from build123d import *

# Parameters (mm, degrees)
SALIENTE_EXTRUIR2_DEPTH = 3
CROQUIS2_W              = 3
CROQUIS2_H              = 10
SALIENTE_EXTRUIR3_DEPTH = 3
CROQUIS3_W              = 10
CROQUIS3_H              = 3
SALIENTE_EXTRUIR4_DEPTH = 3


with BuildPart() as part:
    # Croquis1 → Saliente-Extruir2 (new body)
    with BuildSketch(Plane.XY):
        Polygon((19, -9), (-19, -9), (-19, 9), (-1.5, 9), (-1.5, 6), (-3, 6), (-3, 3), (3, 3), (3, 6), (1.5, 6), (1.5, 9), (19, 9), align=None)
    extrude(amount=SALIENTE_EXTRUIR2_DEPTH)

    # Croquis2 → Saliente-Extruir3 (add)
    with BuildSketch(Plane(origin=(19, 0, 0), x_dir=(0, 0, -1), z_dir=(1, 0, 0))):
        with Locations((-1.5, 0)):
            Rectangle(CROQUIS2_W, CROQUIS2_H)
    saliente_extruir3 = extrude(amount=SALIENTE_EXTRUIR3_DEPTH)

    # Croquis3 → Saliente-Extruir4 (add)
    with BuildSketch(Plane(origin=(0, 9, 0), x_dir=(1, 0, 0), z_dir=(0, 1, 0))):
        with Locations((14.325, -1.5)):
            Rectangle(CROQUIS3_W, CROQUIS3_H)
    saliente_extruir4 = extrude(amount=SALIENTE_EXTRUIR4_DEPTH)

    # Simetría1: Saliente-Extruir3 across plane
    add(saliente_extruir3.mirror(Plane(origin=(0, 0, 0), x_dir=(0, 0, 1), z_dir=(1, 0, 0))))

    # Simetría2: Saliente-Extruir4 across plane
    add(saliente_extruir4.mirror(Plane(origin=(0, 0, 0), x_dir=(0, 0, 1), z_dir=(1, 0, 0))))


solid = part.part
Read the model definition and answer for the solid it produces. Units are mm, in the model's axes. A direction names the side the tool comes from. Give positions to 0.01 mm unless a question says otherwise; leave off trailing zeros. Write each loop counter-clockwise with the first axis right and the second up, starting at its lowest first coordinate (ties: lowest second). Pieces come first, ordered by that corner, then holes. Notation, with made-up numbers: M 13,38 L 20,38 A10 cw 20,51 Z; hole C -33,27.5 d10. An arc over 180 degrees is marked long. One line per item, written item: value. Start each with the question number.
(1) Find the intervals of material crossed by line 1 (X direction, y = 5.5, z = 1.3); line 2 (X direction, y = 6.25, z = 1); line 3 (Y direction, x = 2, z = 0.65), in increasing order.
(2) Find section C-C (x = 5.5). Determine the outline of the cut face in (y, z), plus the area to 3 significant figures.
(3) Find section A-A (y = 6.5). Determine the outline of the cut face in (x, z).
(4) A tool of negligible diameter and unlimited length cuts with its end or side. For faces 5 (the flat face through (-9.325, 10, 2)), 6 (the flat face through (-2, 6, 1)), 7 (the flat face through (19.325, 10, 2)), from which of +Z, -Z, +X, -X, +Y, -Y can it reach the whole face along a straight path? Write none if from no direction.
(5) Find section B-B (z = 2.4). Determine the outline of the cut face in (x, y) (3 decimals).
(6) Find section D-D (y = -6.25). Determine the outline of the cut face in (x, z), plus the area to 3 significant figures.
(7) Flat-ended cylindrical pins translate along their axes: pin 1 Ø1.5 at (y, z) = (11, 2) entering from +X (3 decimals); pin 2 Ø1.5 at (x, z) = (-21, 1) entering from +Y; pin 3 Ø1 at (y, z) = (-6.5, 1.5) entering from -X. Find the tip coordinate at first contact, or state that the pin passes through.
(8) Determine the mould class of faces 1 (the flat face through (-19.325, 10, 2)), 2 (the flat face through (9.325, 10, 2)), 3 (the flat face through (2, 6, 1)), 4 (the flat face through (22, 0, 2)) for opening direction X: pulls with the +X half, pulls with the -X half, needs draft (parallel to the pull), parting line crosses it, or undercut.
Results below:
1. line 1: x = -19 to -3, 3 to 19
1. line 2: x = -19 to -1.5, 1.5 to 19
1. line 3: y = -9 to 3, 6 to 9
2. outline: M -9,0 L 9,0 L 9,3 L -9,3 Z
2. area: 54.0 mm^2
3. outline: M -19,0 L -1.5,0 L -1.5,3 L -19,3 Z; M 1.5,0 L 19,0 L 19,3 L 1.5,3 Z
4. face 5: +Z, -Z, +Y
4. face 6: +Z, -Z
4. face 7: +Z, -Z, +X, +Y
5. outline: M -22,-5 L -19,-5 L -19,-9 L 19,-9 L 19,-5 L 22,-5 L 22,5 L 19,5 L 19,9 L 19.325,9 L 19.325,12 L 9.325,12 L 9.325,9 L 1.5,9 L 1.5,6 L 3,6 L 3,3 L -3,3 L -3,6 L -1.5,6 L -1.5,9 L -9.325,9 L -9.325,12 L -19.325,12 L -19.325,9 L -19,9 L -19,5 L -22,5 Z
6. outline: M -19,0 L 19,0 L 19,3 L -19,3 Z
6. area: 114 mm^2
7. pin 1: stops at x = 19.325
7. pin 2: stops at y = 5
7. pin 3: stops at x = -19
8. face 1: pulls with the -X half
8. face 2: undercut
8. face 3: undercut
8. face 4: pulls with the +X half
